Part model, mm, in its own coordinate system. Face numbers are marked on the shaded views. A direction names the side the tool comes from. Give positions to 0.01 mm unless a question says otherwise; leave off trailing zeros. Order: outer loops, then holes, each group sorted by start corner. A loop starts at its lowest first (then second) coordinate and runs counter-clockwise, first axis right, second up.
1. Drop flat-ended pins along their axis: pin 1 Ø1.5 at (y, z) = (22.5, -16.5) entering from +X; pin 2 Ø10 at (y, z) = (10, -76) entering from +X; pin 3 Ø3 at (x, y) = (2.5, 8) entering from +Z. Give the stop position or say it passes through.
2. Slice it at B-B on y = 8.5. List the corners of the cut face in (x, z).
3. Slice it at D-D on y = 26.5. List the corners of the cut face in (x, z).
4. Probe line 1 (X direction, y = 28, z = 0); line 2 (Z direction, x = 88, y = 16.5); line 3 (Z direction, x = 108, y = 34.5). List the from-to ranges inside material, lowest first.
5. Mould opens along Z. For the marked faces 3, 4 and 5 say: +Z half, -Z half, draft (parallel to the pull), parting line (faces both ways), or undercut.
6. Which spindle directions (+Z, -Z, +X, -X, +Y, -Y) get a long thin tool onto all of the face, cutting with end or side? Do the marked faces 1 and 2. Say none if no direction does.
7. Slice it at A-A on z = 0. List the corners of the cut face in (x, y).
8. Slice it at C-C on x = -5. List the corners of the cut face in (y, z).
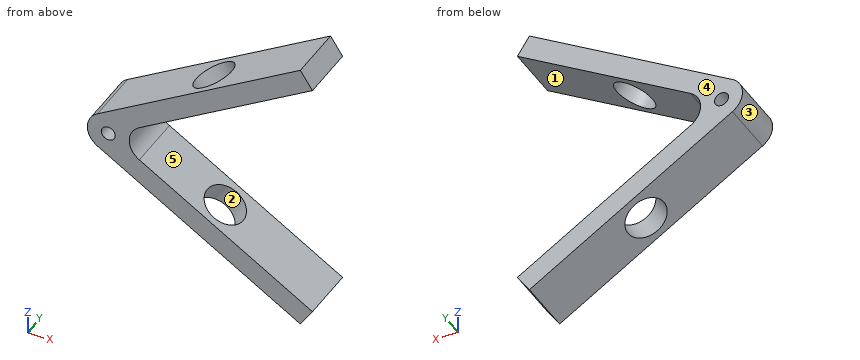
from build123d import *

# Parameters (mm, degrees)
SKETCH1_R           = 5
BOSS_EXTRUDE1_DEPTH = 40
SKETCH2_R           = 15
CUT_EXTRUDE1_DEPTH  = 40
SKETCH3_R           = 15
CUT_EXTRUDE2_DEPTH  = 40


with BuildPart() as part:
    # Sketch1 → Boss-Extrude1 (new body)
    with BuildSketch(Plane(origin=(0, 0, 0), x_dir=(1, 0, 0), z_dir=(0, 1, 0))):
        with BuildLine():
            Line((-37.328010775, 12.814518474), (107.903198598, 101.176817132))
            Line((107.903198598, 101.176817132), (116.545667808, 88.182361447))
            Line((116.545667808, 88.182361447), (-7.328010775, 12.814518474))
            ThreePointArc((-7.328010775, 12.814518474), (-14.531337364, 0), (-7.328010775, -12.814518474))
            Line((-7.328010775, -12.814518474), (116.545667808, -88.182361447))
            Line((116.545667808, -88.182361447), (107.903198598, -101.176817132))
            Line((107.903198598, -101.176817132), (-37.328010775, -12.814518474))
            ThreePointArc((-37.328010775, -12.814518474), (-44.531337364, 0), (-37.328010775, 12.814518474))
        make_face()
        with Locations(Location((-29.531337364, 0, 0), (0, 0, 270))):
            Circle(SKETCH1_R, mode=Mode.SUBTRACT)
    extrude(amount=BOSS_EXTRUDE1_DEPTH)

    # Sketch2 → Cut-Extrude1 (cut)
    with BuildSketch(Plane(origin=(-15.775137276, 0, 25.927825547), x_dir=(0.8543012316036261, 0, 0.5197782274013867), z_dir=(-0.5197782274013867, 0, 0.8543012316036263))):
        with Locations((59.771342119, 20)):
            Circle(SKETCH2_R)
    extrude(amount=-CUT_EXTRUDE1_DEPTH, mode=Mode.SUBTRACT)

    # Sketch3 → Cut-Extrude2 (cut)
    with BuildSketch(Plane(origin=(-15.775137276, 0, -25.927825547), x_dir=(-0.8543012316036261, 0, 0.5197782274013867), z_dir=(-0.5197782274013867, 0, -0.8543012316036263))):
        with Locations((-59.771342119, 20)):
            Circle(SKETCH3_R)
    extrude(amount=-CUT_EXTRUDE2_DEPTH, mode=Mode.SUBTRACT)


solid = part.part
Data:
1. pin 1: stops at x = -0.04
1. pin 2: stops at x = 104.74
1. pin 3: stops at z = 37.96
2. outline: (-37.33, -12.81) - (27.06, -51.99) - (35.17, -38.67) - (-7.33, -12.81) arc R15 cw to (-7.33, 12.81) - (35.17, 38.67) - (27.06, 51.99) - (-37.33, 12.81) arc R15 ccw to start; (43.52, -62) - (107.9, -101.18) - (116.55, -88.18) - (51.62, -48.68) - close; (43.52, 62) - (51.62, 48.68) - (116.55, 88.18) - (107.9, 101.18) - close; hole circle Ø10 at (-29.53, 0)
3. outline: (-37.33, -12.81) - (23.74, -49.97) - (31.84, -36.65) - (-7.33, -12.81) arc R15 cw to (-7.33, 12.81) - (31.84, 36.65) - (23.74, 49.97) - (-37.33, 12.81) arc R15 ccw to start; (46.84, -64.02) - (107.9, -101.18) - (116.55, -88.18) - (54.94, -50.7) - close; (46.84, 64.02) - (54.94, 50.7) - (116.55, 88.18) - (107.9, 101.18) - close; hole circle Ø10 at (-29.53, 0)
4. line 1: x = -44.53 to -34.53, -24.53 to -14.53
4. line 2: z = -89.07 to -70.81, 70.81 to 89.07
4. line 3: z = -101.03 to -82.98, 82.98 to 101.03
5. face 3: parting line
5. face 4: draft
5. face 5: undercut
6. face 1: +X, +Y, -Y
6. face 2: none
7. outline: (-44.53, 0) - (-34.53, 0) - (-34.53, 40) - (-44.53, 40) - close; (-24.53, 0) - (-14.53, 0) - (-14.53, 40) - (-24.53, 40) - close
8. outline: (0, -32.48) - (40, -32.48) - (40, -14.23) - (0, -14.23) - close; (0, 14.23) - (40, 14.23) - (40, 32.48) - (0, 32.48) - close
